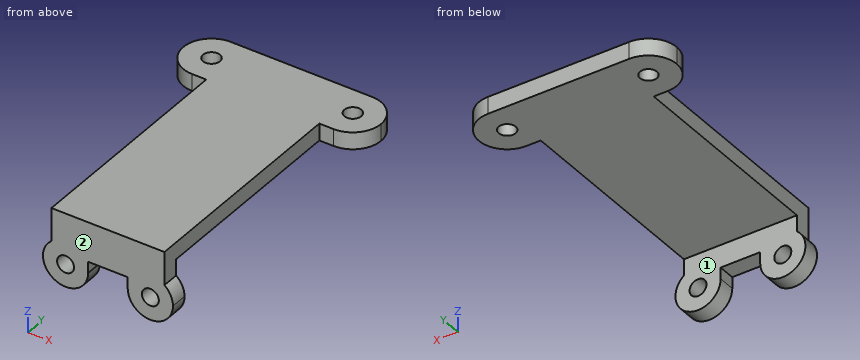
from build123d import *

# Parameters (mm, degrees)
F0_R     = 1.5
F1_DEPTH = 3
F2_W     = 20
F2_H     = 40
F2_R     = 1.5
F2_H_2   = 10
F3_DEPTH = 3


with BuildPart() as f1:
    # F0 (on Front) → F1 (new body)
    with BuildSketch(Plane.XZ):
        with BuildLine():
            Line((10, 2), (-10, 2))
            Line((-10, 2), (-10, -0.8775010008))
            ThreePointArc((-10, -0.8775010008), (-6.7601527307, -0.0690171689), (-4.0358983849, -2))
            Line((-4.0358983849, -2), (-3.5015512196, -2))
            Line((-3.5015512196, -2), (3.5, -2))
            Line((3.5, -2), (4.0358983849, -2))
            ThreePointArc((4.0358983849, -2), (6.7601527307, -0.0690171689), (10, -0.8775010008))
            Line((10, -0.8775010008), (10, 2))
        make_face()
        with BuildLine():
            ThreePointArc((-4.0358983849, -2), (-6.7601527307, -0.0690171689), (-10, -0.8775010008))
            Line((-10, -0.8775010008), (-10, -2))
            Line((-10, -2), (-4.0358983849, -2))
        make_face()
        with BuildLine():
            Line((-10, -2), (-10, -0.8775010008))
            ThreePointArc((-10, -0.8775010008), (-9.282089766, -7.5810830856), (-3.5015512196, -4.1113882884))
            Line((-3.5015512196, -4.1113882884), (-3.5015512196, -3.8886117116))
            ThreePointArc((-3.5015512196, -3.8886117116), (-3.6510874067, -2.9110225671), (-4.0358983849, -2))
            Line((-4.0358983849, -2), (-10, -2))
        make_face()
        with Locations((-7.5, -4)):
            Circle(F0_R, mode=Mode.SUBTRACT)
        with BuildLine():
            ThreePointArc((11.5, -4), (11.1055512755, -2.2679491924), (10, -0.8775010008))
            Line((10, -0.8775010008), (10, -2))
            Line((10, -2), (4.0358983849, -2))
            ThreePointArc((4.0358983849, -2), (3.6362966948, -2.9647238196), (3.5, -4))
            ThreePointArc((3.5, -4), (7.5, -8), (11.5, -4))
        make_face()
        with Locations((7.5, -4)):
            Circle(F0_R, mode=Mode.SUBTRACT)
        with BuildLine():
            Line((10, -2), (10, -0.8775010008))
            ThreePointArc((10, -0.8775010008), (6.7601527307, -0.0690171689), (4.0358983849, -2))
            Line((4.0358983849, -2), (10, -2))
        make_face()
        with BuildLine():
            Line((-3.5015512196, -2), (-4.0358983849, -2))
            ThreePointArc((-4.0358983849, -2), (-3.6510874067, -2.9110225671), (-3.5015512196, -3.8886117116))
            Line((-3.5015512196, -3.8886117116), (-3.5015512196, -2))
        make_face()
        with BuildLine():
            Line((-3.5015512196, -3.8886117116), (-3.5015512196, -4.1113882884))
            ThreePointArc((-3.5015512196, -4.1113882884), (-3.5003878237, -4.0556995446), (-3.5, -4))
            ThreePointArc((-3.5, -4), (-3.5003878237, -3.9443004554), (-3.5015512196, -3.8886117116))
        make_face()
        with BuildLine():
            ThreePointArc((3.5, -4), (3.6362966948, -2.9647238196), (4.0358983849, -2))
            Line((4.0358983849, -2), (3.5, -2))
            Line((3.5, -2), (3.5, -4))
        make_face()
    extrude(amount=F1_DEPTH)

    # F2 (on face) → F3 (join)
    with BuildSketch(Plane.XY.offset(2)):
        with Locations((0, 17)):
            Rectangle(F2_W, F2_H)
        with BuildLine():
            Line((-12.5, 37), (-10, 37))
            Line((-10, 37), (-10, 47))
            Line((-10, 47), (-12.5, 47))
            ThreePointArc((-12.5, 47), (-16.0355339059, 45.5355339059), (-17.5, 42))
            ThreePointArc((-17.5, 42), (-16.0355339059, 38.4644660941), (-12.5, 37))
        make_face()
        with Locations((-12.5, 42)):
            Circle(F2_R, mode=Mode.SUBTRACT)
        with Locations((0, 42)):
            Rectangle(F2_W, F2_H_2)
        with BuildLine():
            Line((10, 47), (10, 37))
            Line((10, 37), (12.5, 37))
            ThreePointArc((12.5, 37), (16.0355339059, 38.4644660941), (17.5, 42))
            ThreePointArc((17.5, 42), (16.0355339059, 45.5355339059), (12.5, 47))
            Line((12.5, 47), (10, 47))
        make_face()
        with Locations((12.5, 42)):
            Circle(F2_R, mode=Mode.SUBTRACT)
    extrude(amount=F3_DEPTH)


solid = f1.part
Model file for the job. Use its own axes, mm. Face numbers are marked on the shaded views. A direction names the side the tool comes from. Coordinates: 2 decimals unless noted, no trailing zeros. Write each loop counter-clockwise with the first axis right and the second up, starting at its lowest first coordinate (ties: lowest second). Pieces come first, ordered by that corner, then holes. Notation, with made-up numbers: (-14, -18) -> (-9, -18) arc R17 ccw to (-9, -6) -> close; hole circle Ø7 at (7.5, 35). An arc over 180 degrees is marked (long way). One line per item, written item: value. Start each with the question number.
1) Which spindle directions (+Z, -Z, +X, -X, +Y, -Y) get a long thin tool onto all of the face, cutting with end or side? Do the marked faces 1 and 2. Say none if no direction does.
2) Slice it at D-D on y = 25.5. Write the cut outline in (x, z).
3) Slice it at C-C on z = -7. Write the cut outline in (x, y).
4) Slice it at B-B on y = 42.5. Write the cut outline in (x, z), then the cut area to 3 significant figures.
5) Slice it at A-A on x = -7.5. Write the cut outline in (y, z), then the cut area to 3 significant figures.
6) Probe probe 1 along Z at (x, y) = (-7.5, -1.25); probe 2 along Y at (x, z) = (-12.5, 3.7); probe 3 along Y at (x, z) = (-9.5, -4.5). List the from-to ranges inside material, lowest first.
7) Flat gauge pins, fed straight in: pin 1 Ø1.8 at (y, z) = (26.5, 3) entering from +X; pin 2 Ø3 at (x, z) = (12, 3.5) entering from -Y; pin 3 Ø4 at (x, z) = (-12.5, -1.5) entering from +Y. Where does each tip first touch, or does it go through?
Answers follow:
1. face 1: -Z, +X, -X, +Y
1. face 2: +Z, -Z, +X, -X, -Y
2. outline: (-10, 2) -> (10, 2) -> (10, 5) -> (-10, 5) -> close
3. outline: (-10.15, -3) -> (-4.85, -3) -> (-4.85, 0) -> (-10.15, 0) -> close; (4.85, -3) -> (10.15, -3) -> (10.15, 0) -> (4.85, 0) -> close
4. outline: (-17.47, 2) -> (-13.91, 2) -> (-13.91, 5) -> (-17.47, 5) -> close; (-11.09, 2) -> (11.09, 2) -> (11.09, 5) -> (-11.09, 5) -> close; (13.91, 2) -> (17.47, 2) -> (17.47, 5) -> (13.91, 5) -> close
4. area: 87.9 mm2
5. outline: (-3, -8) -> (0, -8) -> (0, -5.5) -> (-3, -5.5) -> close; (-3, -2.5) -> (0, -2.5) -> (0, 2) -> (47, 2) -> (47, 5) -> (-3, 5) -> close
5. area: 171 mm2
6. probe 1: -8 to -5.5, -2.5 to 5
6. probe 2: 37 to 40.5, 43.5 to 47
6. probe 3: -3 to 0
7. pin 1: x = 10
7. pin 2: y = 37
7. pin 3: y = 0
